```python
from build123d import *

# Parameters (mm, degrees)
MODEL_R             = 1.3
MODEL_R_2           = 3.74995
BOSS_EXTRUDE1_DEPTH = 3


with BuildPart() as part:
    # Model → Boss-Extrude1 (new body)
    with BuildSketch(Plane.XY):
        with BuildLine():
            Line((59.647938224, 46.456741559), (50.84903604, 26.016099779))
            ThreePointArc((50.84903604, 26.016099779), (52.941556865, 20.760497372), (58.197159265, 22.8530182))
            Line((58.197159265, 22.8530182), (66.996061448, 43.293659979))
            ThreePointArc((66.996061448, 43.293659979), (68.276182261, 45.464386961), (70.05834452, 47.246145252))
            ThreePointArc((70.05834452, 47.246145252), (68.756948833, 57.501076502), (60.413932787, 51.397689825))
            ThreePointArc((60.413932787, 51.397689825), (60.344733109, 48.87856769), (59.647938224, 46.456741559))
        make_face()
        with Locations((54.523097656, 24.434558988)):
            Circle(MODEL_R, mode=Mode.SUBTRACT)
        with Locations((66.384679731, 51.989955386)):
            Circle(MODEL_R_2, mode=Mode.SUBTRACT)
        with BuildLine():
            Line((63.349317004, 42.409481853), (61.372391017, 37.816904838))
            ThreePointArc((61.372391017, 37.816904838), (60.058490416, 37.293774632), (59.535360211, 38.607675233))
            Line((59.535360211, 38.607675233), (61.512286198, 43.200252248))
            ThreePointArc((61.512286198, 43.200252248), (62.826186798, 43.723382454), (63.349317004, 42.409481853))
        make_face(mode=Mode.SUBTRACT)
    extrude(amount=BOSS_EXTRUDE1_DEPTH)


solid = part.part
```
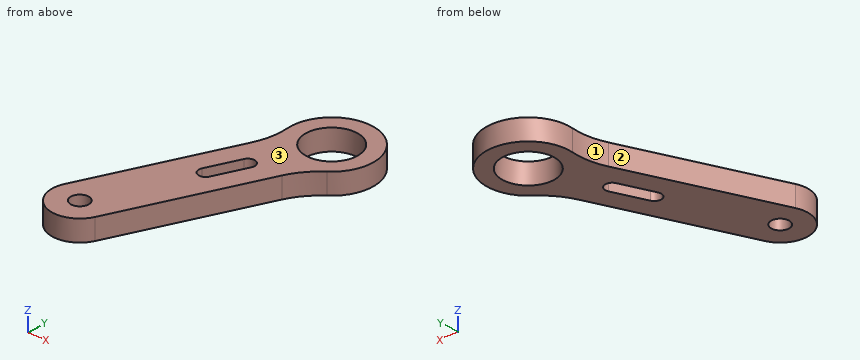
Verification items for the finished model (mm, model axes). Face numbers are marked on the shaded views. Coordinates: 2 decimals unless noted, no trailing zeros. Write each loop counter-clockwise with the first axis right and the second up, starting at its lowest first coordinate (ties: lowest second). Pieces come first, ordered by that corner, then holes. Notation, with made-up numbers: M 27.25,69 L 60.25,69 A14 ccw 60.25,96 Z; hole C -13.5,-0.75 d5. An arc over 180 degrees is marked long. Answer as a JSON object with one key per item and string values. Group by question number.
(1) Cross-section at A-A, the plane x = 69.5. Record the cut outline in (y, z), and give its area (3 significant figures).
(2) Material ranges on line 1 (Y direction, x = 63, z = 0.3); line 2 (Y direction, x = 69, z = 2.1); line 3 (Y direction, x = 68, z = 1.75), recorded low to high.
(3) Cross-section at C-C, the plane y = 41. Record the cut outline in (x, z), and give its area (3 significant figures).
(4) Gauge pin test, flat ends, axial feed: pin 1 (12 mm diameter, centred on x = 60.5, y = 42.5, fed in from -Z); pin 2 (1 mm diameter, centred on y = 41, z = 2.5, fed in from -X). Record the tip position at first contact, or that the pin passes through.
(5) Cross-section at B-B, the plane z = 2.3. Record the cut outline in (x, y).
(6) Cross-section at D-D, the plane x = 57. Record the cut outline in (y, z).
(7) Release check for a two-part mould opening along Y. For the marked faces 1, 2 and 3 record: +Y half, -Y half, draft (parallel to the pull), parting line (faces both ways), or undercut.
Reply:
{
 "1": {"outline": "M 46.78,0 L 49.9,0 L 49.9,3 L 46.78,3 Z; M 54.08,0 L 57.12,0 L 57.12,3 L 54.08,3 Z", "area": "18.5 mm²"},
 "2": {"line 1": "34.01 to 41.6, 43.63 to 50.38, 53.6 to 56.94", "line 2": "46.3 to 49.3, 54.68 to 57.39", "line 3": "45.09 to 48.61, 55.37 to 57.77"},
 "3": {"outline": "M 57.3,0 L 60.57,0 L 60.57,3 L 57.3,3 Z; M 62.74,0 L 66.01,0 L 66.01,3 L 62.74,3 Z", "area": "19.6 mm²"},
 "4": {"pin 1": "z = 0", "pin 2": "x = 57.08"},
 "5": {"outline": "M 50.85,26.02 A4 ccw 58.2,22.85 L 67,43.29 A10 cw 70.06,47.25 A6 ccw long 60.41,51.4 A10 cw 59.65,46.46 Z; hole C 54.52,24.43 d2.6; hole M 59.54,38.61 A1 ccw 61.37,37.82 L 63.35,42.41 A1 ccw 61.51,43.2 Z; hole C 66.38,51.99 d7.5"},
 "6": {"outline": "M 21.29,0 L 40.31,0 L 40.31,3 L 21.29,3 Z"},
 "7": {"face 1": "undercut", "face 2": "+Y half", "face 3": "draft"}
}
